Geometry: final body of the model. Coordinates: model frame, mm. Face numbers are marked on the shaded views. A direction names the side the tool comes from. Give positions to 0.01 mm unless a question says otherwise; leave off trailing zeros. Write each loop counter-clockwise with the first axis right and the second up, starting at its lowest first coordinate (ties: lowest second). Pieces come first, ordered by that corner, then holes.
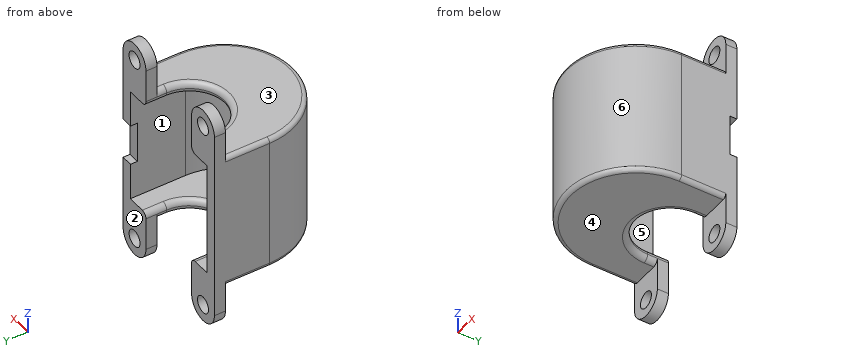
```python
from build123d import *

# Parameters (mm, degrees)
BASE_DEPTH              = 8
CROQUIS5_R              = 6
PERFORACIONES_DEPTH     = 8
SALIENTE_EXTRUIR5_DEPTH = 100
VACIADO2_START          = -112
VACIADO2_DEPTH          = 84
CORTAR_EXTRUIR3_DEPTH   = 100
CROQUIS10_W             = 8
CROQUIS10_H             = 30
CORTAR_EXTRUIR4_DEPTH   = 5
REDONDEO1_R             = 4
REDONDEO2_R             = 4
REDONDEO3_R             = 3


# Read off the part's stored shape, not the designer's step: Vaciado2
with BuildPart() as part:
    # Croquis4 → Base (new body)
    with BuildSketch(Plane(origin=(0, 0, 0), x_dir=(1, 0, 0), z_dir=(0, 1, 0))):
        with BuildLine():
            Line((0, 0), (0, 140))
            ThreePointArc((0, 140), (-12.5, 152.5), (-25, 140))
            Line((-25, 140), (-25, 120))
            Line((-25, 120), (-75, 120))
            Line((-75, 120), (-75, 140))
            ThreePointArc((-75, 140), (-87.5, 152.5), (-100, 140))
            Line((-100, 140), (-100, 0))
            ThreePointArc((-100, 0), (-87.5, -12.5), (-75, 0))
            Line((-75, 0), (-75, 20))
            Line((-75, 20), (-25, 20))
            Line((-25, 20), (-25, 0))
            ThreePointArc((-25, 0), (-12.5, -12.5), (0, 0))
        make_face()
    extrude(amount=BASE_DEPTH)

    # Croquis5 → Perforaciones (cut)
    with BuildSketch(Plane.XZ):
        with Locations(Location((-87.5, 0, 0), (0, 0, 270))):
            Circle(CROQUIS5_R)
        with Locations(Location((-12.5, 0, 0), (0, 0, 270))):
            Circle(CROQUIS5_R)
        with Locations(Location((-87.5, -140, 0), (0, 0, 270))):
            Circle(CROQUIS5_R)
        with Locations(Location((-12.5, -140, 0), (0, 0, 270))):
            Circle(CROQUIS5_R)
    extrude(amount=-PERFORACIONES_DEPTH, mode=Mode.SUBTRACT)

    # Croquis7 → Saliente-Extruir5 (add)
    with BuildSketch(Plane.XY.offset(-20)):
        with BuildLine():
            Line((-100, 0), (-100, -32))
            ThreePointArc((-100, -32), (-50, -82), (0, -32))
            Line((0, -32), (0, 0))
            Line((0, 0), (-100, 0))
        make_face()
    extrude(amount=-SALIENTE_EXTRUIR5_DEPTH)

    # Vaciado2 outline → Vaciado2 (cut)
    with BuildSketch(Plane.XY.offset(VACIADO2_START)):
        with BuildLine():
            Line((-8, -32), (-8, 8))
            Line((-8, 8), (-92, 8))
            Line((-92, 8), (-92, -32))
            ThreePointArc((-92, -32), (-50, -74), (-8, -32))
        make_face()
    extrude(amount=VACIADO2_DEPTH, mode=Mode.SUBTRACT)

    # Croquis9 → Cortar-Extruir3 (cut)
    with BuildSketch(Plane.XY.offset(-20)):
        with BuildLine():
            Line((-75, 8), (-75, -7))
            ThreePointArc((-75, -7), (-50, -32), (-25, -7))
            Line((-25, -7), (-25, 8))
            Line((-25, 8), (-75, 8))
        make_face()
    extrude(amount=-CORTAR_EXTRUIR3_DEPTH, mode=Mode.SUBTRACT)

    # Croquis10 → Cortar-Extruir4 (cut)
    with BuildSketch(Plane(origin=(0, 8, 0), x_dir=(1, 0, 0), z_dir=(0, 1, 0))):
        with Locations((-4, 70)):
            Rectangle(CROQUIS10_W, CROQUIS10_H)
    extrude(amount=-CORTAR_EXTRUIR4_DEPTH, mode=Mode.SUBTRACT)

    # Redondeo1
    redondeo1_edges = [part.edges().sort_by_distance(p)[0] for p in [
        (-75, 0.5, -28),
        (-50, -32, -28),
        (-25, 0.5, -28),
        (-75, -3.5, -20),
        (-25, -3.5, -20),
    ]]
    fillet(redondeo1_edges, radius=REDONDEO1_R - 0.0001)  # a hair under: the kernel refuses the full size

    # Redondeo2
    redondeo2_edges = [part.edges().sort_by_distance(p)[0] for p in [
        (-25, 0.5, -112),
        (-25, -3.5, -120),
        (-50, -32, -112),
        (-75, 0.5, -112),
        (-75, -3.5, -120),
    ]]
    fillet(redondeo2_edges, radius=REDONDEO2_R - 0.0001)  # a hair under: the kernel refuses the full size

    # Redondeo3
    redondeo3_edges = [part.edges().sort_by_distance(p)[0] for p in [
        (0, -16, -120),
        (-50, -82, -120),
        (-100, -16, -120),
        (-100, -16, -20),
        (-50, -82, -20),
        (0, -16, -20),
    ]]
    fillet(redondeo3_edges, radius=REDONDEO3_R)


solid = part.part
```
Item 1: Section C-C, the plane x = -12.5. State how many separate pieces and enclosed holes the cut face has, plus the area to 3 significant figures.
Found:
separate pieces: 3
enclosed holes: 0
area: 2,680 mm2
Item 2: Line query: L1, parallel to Z at x = -87, y = 3; L2, parallel to Z at x = -87.5, y = -23; L3, parallel to Z at x = -22, y = -2. Output: solid intervals per line, ascending.
Found:
L1: z = -152.49 to -145.98, -134.02 to -112, -28 to -5.98, 5.98 to 12.49
L2: z = -120 to -112, -28 to -20
L3: z = -119.87 to -112.13, -27.87 to -20.13
Item 3: Pin query (flat end, axial travel): pin 1 Ø8 at (x, z) = (-48, -122) entering from +Y; pin 2 Ø2 at (x, z) = (-76, -103.5) entering from +Y; pin 3 Ø20 at (x, z) = (-90, -4.5) entering from -Y. Return the tip coordinate at first contact, or that it passes through.
Found:
pin 1: stops at y = -32.43
pin 2: stops at y = -64.17
pin 3: stops at y = 0
Item 4: Pull-direction query (Z, two-part tool) for the marked faces 3, 4, 5 and 6; classes: +Z half, -Z half, draft (parallel to the pull), parting line (faces both ways), or undercut.
Found:
face 3: +Z half
face 4: -Z half
face 5: undercut
face 6: draft
Item 5: Section A-A, the plane z = -12. Return the cut outline in (x, y).
Found:
outline: (-100, 0) - (-75, 0) - (-75, 8) - (-100, 8) - close; (-25, 0) - (0, 0) - (0, 8) - (-25, 8) - close
Item 6: Section B-B, the plane z = -102. Return the cut outline in (x, y), plus the area to 3 significant figures.
Found:
outline: (-100, -32) arc R50 ccw to (0, -32) - (0, 8) - (-8, 8) - (-8, -32) arc R42 cw to (-92, -32) - (-92, 8) - (-100, 8) - close
area: 1,800 mm2
Item 7: Reachability of the marked faces 1 and 2 from +Z, -Z, +X, -X, +Y, -Y: full face, straight path, thin tool, end or side. Return the list, or none.
Found:
face 1: +Y
face 2: +Z, -Z, +X, -X, +Y
